from build123d import *

# Parameters (mm, degrees)
SKETCH6_R               = 6
BOSS_EXTRUDE4_DEPTH     = 2.5
SKETCH7_R               = 6.1
BOSS_EXTRUDE5_DEPTH     = 5.2
SKETCH8_R               = 6.05
BOSS_EXTRUDE6_DEPTH     = 5.2
SKETCH13_R              = 10
BOSS_EXTRUDE7_DEPTH     = 5
CUT_EXTRUDE1_DEPTH      = 6.2
CUT_EXTRUDE1_DEPTH_BACK = 11.2
CHAMFER1_SIZE           = 0.5


with BuildPart() as part:
    # Sketch6 → Boss-Extrude4 (new body, symmetric)
    with BuildSketch(Plane.XY):
        Circle(SKETCH6_R)
    extrude(amount=BOSS_EXTRUDE4_DEPTH, both=True)

    # Sketch7 → Boss-Extrude5 (add)
    with BuildSketch(Plane.XY.offset(2.5)):
        with Locations((0, 1)):
            Circle(SKETCH7_R)
    extrude(amount=BOSS_EXTRUDE5_DEPTH)

    # Sketch8 → Boss-Extrude6 (add)
    with BuildSketch(Plane(origin=(0, 0, -2.5), x_dir=(-1, 0, 0), z_dir=(0, 0, -1))):
        with Locations((0, -1)):
            Circle(SKETCH8_R)
    extrude(amount=BOSS_EXTRUDE6_DEPTH)

    # Sketch13 → Boss-Extrude7 (add)
    with BuildSketch(Plane.XY.offset(2.5)):
        Circle(SKETCH13_R)
    extrude(amount=-BOSS_EXTRUDE7_DEPTH)

    # Sketch11 → Cut-Extrude1 (cut, two sides)
    with BuildSketch(Plane.XY.offset(2.5)) as cut_extrude1_sk:
        with BuildLine():
            Line((-1.983053202, -2.7), (1.983053202, -2.7))
            ThreePointArc((1.983053202, -2.7), (3.35, 0), (1.983053202, 2.7))
            Line((1.983053202, 2.7), (-1.983053202, 2.7))
            ThreePointArc((-1.983053202, 2.7), (-3.35, 0), (-1.983053202, -2.7))
        make_face()
    extrude(amount=CUT_EXTRUDE1_DEPTH, mode=Mode.SUBTRACT)
    extrude(cut_extrude1_sk.sketch, amount=-CUT_EXTRUDE1_DEPTH_BACK, mode=Mode.SUBTRACT)

    # Chamfer1
    chamfer1_edges = [part.edges().sort_by_distance(p)[0] for p in [
        (6.05, -1, -7.7),
        (-6.1, 1, 7.7),
    ]]
    chamfer(chamfer1_edges, length=CHAMFER1_SIZE)


solid = part.part
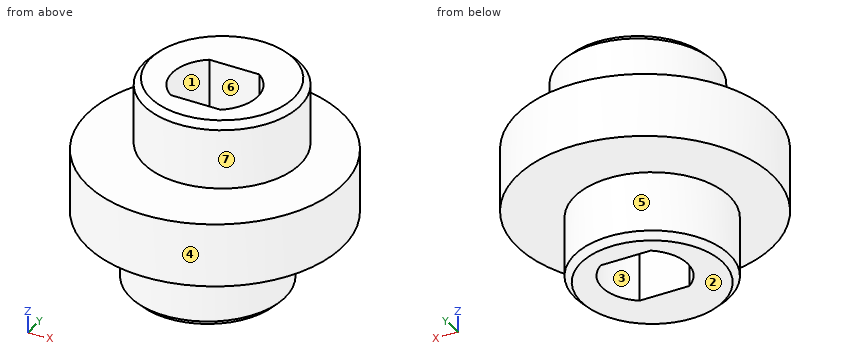
The model under review builds one solid part; all positions refer to its coordinate system, in mm. Face numbers are marked on the shaded views. A direction names the side the tool comes from. Round coordinates to 2 decimals unless told otherwise and drop trailing zeros. Write each loop counter-clockwise with the first axis right and the second up, starting at its lowest first coordinate (ties: lowest second). Pieces come first, ordered by that corner, then holes. Notation, with made-up numbers: M 9.5,-35 L 48.5,-35 A18 cw 48.5,-17 Z; hole C 66,3.5 d2. An arc over 180 degrees is marked long. Use a Markdown table: item, result. Add a question column.
Q1. To check wall thickness, follow line 1 (Z direction, x = -8, y = -1.25); line 2 (Y direction, x = -1.25, z = 4.75); line 3 (Y direction, x = -2.5, z = 7). State the ranges of each line that lie inside material, in increasing order.
Q2. We need section B-B, the plane z = -5. State the section outline as (x, y) points.
Q3. We need section D-D, the plane x = 8.25. State the section outline as (y, z) points, plus the area to 3 significant figures.
Q4. We need section C-C, the plane z = -1.5. State the section outline as (x, y) points, plus the area to 3 significant figures.
Q5. The part is to be moulded in two halves that separate along X. For the marked faces 1, 2, 3 and 4, say which applies: pulls with the +X half, pulls with the -X half, needs draft (parallel to the pull), parting line crosses it, or undercut.
Q6. Insertion check: pin 1 (6 mm diameter, centred on x = 2.5, z = -5, fed in from -Y); pin 2 (1.5 mm diameter, centred on x = 1.5, y = -8, fed in from +Z); pin 3 (2 mm diameter, centred on y = -3.5, z = -1.5, fed in from -X). Each pin has a flat end and moves straight along its axis. Give the tip position at first contact, or say it passes through.
Q7. We need section A-A, the plane x = 0. State the section outline as (y, z) points.
Q8. Machinability: for the marked faces 5, 6 and 7, which of the approach directions +Z, -Z, +X, -X, +Y, -Y give a long, thin tool a straight path to every point of the face, cutting with its end or side? Answer none if there is none.
Findings below:
| question | item | result |
|---|---|---|
| 1 | line 1 | z = -2.5 to 2.5 |
| 1 | line 2 | y = -4.97 to -2.7, 2.7 to 6.97 |
| 1 | line 3 | y = -4.56 to -2.23, 2.23 to 6.56 |
| 2 | outline | C 0,-1 d12.1; hole M -1.98,-2.7 L 1.98,-2.7 A3.35 ccw 1.98,2.7 L -1.98,2.7 A3.35 ccw Z |
| 3 | outline | M -5.65,-2.5 L 5.65,-2.5 L 5.65,2.5 L -5.65,2.5 Z |
| 3 | area | 56.5 mm² |
| 4 | outline | C 0,0 d20; hole M -1.98,-2.7 L 1.98,-2.7 A3.35 ccw 1.98,2.7 L -1.98,2.7 A3.35 ccw Z |
| 4 | area | 282 mm² |
| 5 | face 1 | undercut |
| 5 | face 2 | needs draft |
| 5 | face 3 | undercut |
| 5 | face 4 | parting line crosses it |
| 6 | pin 1 | stops at y = -9.96 |
| 6 | pin 2 | stops at z = 2.5 |
| 6 | pin 3 | stops at x = -9.68 |
| 7 | outline | M -10,-2.5 L -7.05,-2.5 L -7.05,-7.2 L -6.55,-7.7 L -2.7,-7.7 L -2.7,7.7 L -4.6,7.7 L -5.1,7.2 L -5.1,2.5 L -10,2.5 Z; M 2.7,-7.7 L 4.55,-7.7 L 5.05,-7.2 L 5.05,-2.5 L 10,-2.5 L 10,2.5 L 7.1,2.5 L 7.1,7.2 L 6.6,7.7 L 2.7,7.7 Z |
| 8 | face 5 | -Z |
| 8 | face 6 | +Z, -Z |
| 8 | face 7 | +Z |
